Read the model definition and answer for the solid it produces. Units are mm, in the model's axes. A direction names the side the tool comes from. Coordinates: 2 decimals unless noted, no trailing zeros. Loops run counter-clockwise (first coordinate to the right, second up) from the corner with the lowest first, then second, coordinate; pieces in that order, holes last.
Q1. Straight lines are drawn through the part: line 1 (X direction, y = 2.35, z = 12); line 2 (Y direction, x = 15, z = -2.25); line 3 (X direction, y = 87.8, z = 0.25). For each, find the intervals that lie inside material, in ascending order.
Q2. The mould has two halves that part along Y. Classify faces 1 (the face through (-10, 2, 15)), 2 (the face through (-10, 0, 0)), 3 (the face through (-11.75, 85, -1)): pulls with the +Y half, pulls with the -Y half, needs draft (parallel to the pull), parting line crosses it, or undercut.
Q3. Section A-A (x = 14.5) is taken. Give the vertices of the cut face in (y, z), then the cut area to 3 significant figures.
Q4. Section D-D (x = -76.7) is taken. Give the vertices of the cut face in (y, z), then the cut area to 3 significant figures.
Q5. Flat-ended cylindrical pins translate along their axes: P1, Ø13.5, axis at x = 8.5, y = 77.5, coming from the +Z side; P2, Ø3, axis at x = 14.5, z = -12, coming from the -Y side; P3, Ø3, axis at y = 22.5, z = -1.5, coming from the -X side; P4, Ø5, axis at x = 16.5, z = 2.5, coming from the -Y side. Find the tip coordinate at first contact, or state that the pin passes through.
Q6. Section B-B (y = 63) is taken. Give the vertices of the cut face in (x, z), then the cut area to 3 significant figures.
Q7. Which of the six approach directions +Z, -Z, +X, -X, +Y, -Y give full straight-line access (tool end or side, diameter ignored) to faces 4 (the face through (23, 89.8, -1)), 5 (the face through (-10, 68, -12)), 6 (the face through (-11, 3, 7)), 7 (the face through (-9, 91, 6))?
Q8. Section C-C (z = 1.75) is taken. Give the vertices of the cut face in (x, y).
from build123d import *

# Parameters (mm, degrees)
SKETCH_1_W               = 126.3
SKETCH_1_H               = 42.9
SKETCH_1_W_2             = 2
SKETCH_1_W_3             = 62.15
EXTRUDE_6_DEPTH          = 15
SKETCH_2_W               = 62.15
SKETCH_2_H               = 42.9
CUT_EXTRUDE_1_DEPTH      = 23
SKETCH_4_W               = 10
SKETCH_4_H               = 40
CUT_EXTRUDE_2_DEPTH      = 159.899905601
CUT_EXTRUDE_3_DEPTH      = 119.456321064
CUT_EXTRUDE_3_DEPTH_BACK = 119.456321064
SKETCH_5_W               = 10
SKETCH_5_H               = 40
CUT_EXTRUDE_4_DEPTH      = 159.899905601
CUT_EXTRUDE_4_DEPTH_BACK = 159.899905601
SKETCH_6_W               = 9
SKETCH_6_H               = 46.7
SKETCH_7_W               = 14
SKETCH_7_H               = 11.9
CUT_EXTRUDE_5_DEPTH      = 23
SKETCH_9_R               = 1.6
CUT_EXTRUDE_6_DEPTH      = 10
CUT_EXTRUDE_7_DEPTH      = 159.899905601
CUT_EXTRUDE_7_DEPTH_BACK = 159.899905601
SKETCH_11_W              = 3
SKETCH_11_H              = 46.7
SKETCH_14_W              = 7
SKETCH_14_H              = 18
EXTRUDE_8_DEPTH          = 46.7
SKETCH_15_W              = 2.315581883
SKETCH_15_H              = 42.9
SKETCH_15_R              = 1.6
CUT_EXTRUDE_9_DEPTH      = 14
SKETCH_19_W              = 3
SKETCH_19_H              = 18
EXTRUDE_9_DEPTH          = 46.7
SKETCH_20_W              = 140.3
SKETCH_20_H              = 2
EXTRUDE_10_DEPTH         = 18
SKETCH_21_R              = 1.6
CUT_EXTRUDE_13_DEPTH     = 14
SKETCH_23_W              = 2
SKETCH_23_H              = 2
EXTRUDE_11_DEPTH         = 14


with BuildPart() as part:
    # 草图1 → 凸台-拉伸6 (new, symmetric)
    # profile 1 of 4: a face of its own
    with BuildSketch(Plane.XY):
        Polygon((-39.5, 0), (-39.5, 3), (-21.5, 3), (-21.5, 43), (-75.9, 43), (-75.9, 89.7), (54.4, 89.7), (54.4, 43), (0, 43), (0, 3), (18, 3), (18, 0), align=None)
        with Locations((-10.75, 66.35)):
            Rectangle(SKETCH_1_W, SKETCH_1_H, mode=Mode.SUBTRACT)
    # profile 2 of 4: a face of its own
    with BuildSketch(Plane.XY):
        with Locations((-10.75, 66.35)):
            Rectangle(SKETCH_1_W_2, SKETCH_1_H)
    # profile 3 of 4: a face of its own
    with BuildSketch(Plane.XY):
        with Locations((21.325, 66.35)):
            Rectangle(SKETCH_1_W_3, SKETCH_1_H)
    # profile 4 of 4: a face of its own
    with BuildSketch(Plane.XY):
        with Locations((-42.825, 66.35)):
            Rectangle(SKETCH_1_W_3, SKETCH_1_H)
    extrude(amount=EXTRUDE_6_DEPTH, both=True)

    # 草图2 → 切除-拉伸1 (cut)
    with BuildSketch(Plane.XY.offset(15)):
        with Locations((-42.825, 66.35)):
            Rectangle(SKETCH_2_W, SKETCH_2_H)
        with Locations((21.325, 66.35)):
            Rectangle(SKETCH_2_W, SKETCH_2_H)
    extrude(amount=-CUT_EXTRUDE_1_DEPTH, mode=Mode.SUBTRACT)

    # 草图4 → 切除-拉伸2 (cut, through all)
    with BuildSketch(Plane.ZY.offset(75.9)):
        with Locations((10, 23)):
            Rectangle(SKETCH_4_W, SKETCH_4_H)
    extrude(amount=-CUT_EXTRUDE_2_DEPTH, mode=Mode.SUBTRACT)

    # 草图5 → 切除-拉伸3 (cut, two sides: drawn at the far end of the back side and taken through both)
    with BuildSketch(Plane.ZY.offset(21.5).offset(-CUT_EXTRUDE_3_DEPTH_BACK)):
        with Locations((-10, 23)):
            Rectangle(SKETCH_5_W, SKETCH_5_H)
    extrude(amount=CUT_EXTRUDE_3_DEPTH + CUT_EXTRUDE_3_DEPTH_BACK, mode=Mode.SUBTRACT)

    # 草图6 → 切除-拉伸4 (cut, two sides: drawn at the far end of the back side and taken through both)
    with BuildSketch(Plane.ZY.offset(75.9).offset(-CUT_EXTRUDE_4_DEPTH_BACK)):
        with Locations((10.5, 66.35)):
            Rectangle(SKETCH_6_W, SKETCH_6_H)
    extrude(amount=CUT_EXTRUDE_4_DEPTH + CUT_EXTRUDE_4_DEPTH_BACK, mode=Mode.SUBTRACT)

    # 草图7 → 切除-拉伸5 (cut)
    with BuildSketch(Plane.ZY.offset(11.75)):
        with Locations((-1, 73.85)):
            Rectangle(SKETCH_7_W, SKETCH_7_H)
    extrude(amount=-CUT_EXTRUDE_5_DEPTH, mode=Mode.SUBTRACT)

    # 草图9 → 切除-拉伸6 (cut)
    with BuildSketch(Plane.XZ):
        with Locations(Location((-36, 12, 0), (0, 0, 270))):
            Circle(SKETCH_9_R)
        with Locations(Location((-36, -12, 0), (0, 0, 270))):
            Circle(SKETCH_9_R)
        with Locations(Location((14.5, 12, 0), (0, 0, 270))):
            Circle(SKETCH_9_R)
        with Locations(Location((14.5, -12, 0), (0, 0, 270))):
            Circle(SKETCH_9_R)
    extrude(amount=-CUT_EXTRUDE_6_DEPTH, mode=Mode.SUBTRACT)

    # 草图11 → 切除-拉伸7 (cut, two sides: drawn at the far end of the back side and taken through both)
    with BuildSketch(Plane.ZY.offset(75.9).offset(-CUT_EXTRUDE_7_DEPTH_BACK)):
        with Locations((-13.5, 66.35)):
            Rectangle(SKETCH_11_W, SKETCH_11_H)
    extrude(amount=CUT_EXTRUDE_7_DEPTH + CUT_EXTRUDE_7_DEPTH_BACK, mode=Mode.SUBTRACT)

    # 草图14 → 凸台-拉伸8 (add)
    with BuildSketch(Plane(origin=(0, 89.7, 0), x_dir=(1, 0, 0), z_dir=(0, 1, 0))):
        with Locations((57.9, 3)):
            Rectangle(SKETCH_14_W, SKETCH_14_H)
    extrude(amount=-EXTRUDE_8_DEPTH)

    # 草图15 → 切除-拉伸9 (cut)
    with BuildSketch(Plane.XY.offset(6)):
        with BuildLine():
            ThreePointArc((60.11573898, 44.9), (58.51573898, 46.5), (56.91573898, 44.9))
            ThreePointArc((56.91573898, 44.9), (58.51573898, 43.3), (60.11573898, 44.9))
        make_face()
        with Locations((53.557790942, 66.35)):
            Rectangle(SKETCH_15_W, SKETCH_15_H)
        Polygon((52.4, 44.9), (52.4, 87.8), (-9.75, 87.8), (-9.75, 79.8), (-11.75, 79.8), (-11.75, 87.8), (-73.9, 87.8), (-73.9, 44.9), (-11.75, 44.9), (-11.75, 67.9), (-9.75, 67.9), (-9.75, 44.9), align=None)
        with Locations((58.51385679, 87.8)):
            Circle(SKETCH_15_R)
    extrude(amount=-CUT_EXTRUDE_9_DEPTH, mode=Mode.SUBTRACT)

    # 草图19 → 凸台-拉伸9 (add)
    with BuildSketch(Plane(origin=(0, 89.7, 0), x_dir=(1, 0, 0), z_dir=(0, 1, 0))):
        with Locations((-77.4, 3)):
            Rectangle(SKETCH_19_W, SKETCH_19_H)
    extrude(amount=-EXTRUDE_9_DEPTH)

    # 草图20 → 凸台-拉伸10 (add)
    with BuildSketch(Plane.XY.offset(6)):
        with Locations((-8.75, 90.7)):
            Rectangle(SKETCH_20_W, SKETCH_20_H)
    extrude(amount=-EXTRUDE_10_DEPTH)

    # 草图21 → 切除-拉伸13 (cut)
    with BuildSketch(Plane.XY.offset(6)):
        with Locations((-76.7, 44.9)):
            Circle(SKETCH_21_R)
        Polygon((-73.9, 89.8), (-73.9, 87.8), (-11.75, 87.8), (54.715581883, 87.8), (54.715581883, 89.8), align=None)
        with Locations((-76.7, 87.8)):
            Circle(SKETCH_21_R)
    extrude(amount=-CUT_EXTRUDE_13_DEPTH, mode=Mode.SUBTRACT)

    # 草图23 → 凸台-拉伸11 (add)
    with BuildSketch(Plane.XY.offset(-8)):
        with Locations((-10.75, 88.8)):
            Rectangle(SKETCH_23_W, SKETCH_23_H)
    extrude(amount=EXTRUDE_11_DEPTH)


solid = part.part
Numbers:
1. line 1: x = -39.5 to -37.6, -34.4 to 12.9, 16.1 to 18
1. line 2: y = 0 to 3, 43 to 44.9, 89.8 to 91.7
1. line 3: x = -78.9 to -78.3, -75.1 to -73.9, -11.75 to -9.75, 54.72 to 56.91, 60.11 to 61.4
2. face 1: needs draft
2. face 2: pulls with the -Y half
2. face 3: undercut
3. outline: (0, -15) - (3, -15) - (3, -13.6) - (0, -13.6) - close; (0, -10.4) - (3, -10.4) - (3, 10.4) - (0, 10.4) - close; (0, 13.6) - (3, 13.6) - (3, 15) - (0, 15) - close; (43, -12) - (91.7, -12) - (91.7, 6) - (89.8, 6) - (89.8, -8) - (44.9, -8) - (44.9, 6) - (43, 6) - close
3. area: 319 mm2
4. outline: (43, -12) - (91.7, -12) - (91.7, 6) - (89.4, 6) - (89.4, -8) - (86.2, -8) - (86.2, 6) - (46.5, 6) - (46.5, -8) - (43.3, -8) - (43.3, 6) - (43, 6) - close
4. area: 787 mm2
5. P1: stops at z = -8
5. P2: stops at y = 43
5. P3: stops at x = -21.5
5. P4: stops at y = 0
6. outline: (-78.9, -12) - (61.4, -12) - (61.4, 6) - (54.72, 6) - (54.72, -8) - (-9.75, -8) - (-9.75, 6) - (-11.75, 6) - (-11.75, -8) - (-73.9, -8) - (-73.9, 6) - (-78.9, 6) - close
6. area: 753 mm2
7. face 4: +Z
7. face 5: -Z, +X, -X, +Y
7. face 6: none
7. face 7: +Z, +X, -X, +Y
8. outline: (-78.9, 43) - (-21.5, 43) - (-21.5, 3) - (-39.5, 3) - (-39.5, 0) - (18, 0) - (18, 3) - (0, 3) - (0, 43) - (61.4, 43) - (61.4, 91.7) - (-78.9, 91.7) - close; hole circle Ø3.2 at (-76.7, 44.9); hole circle Ø3.2 at (-76.7, 87.8); hole (-73.9, 44.9) - (-11.75, 44.9) - (-11.75, 67.9) - (-9.75, 67.9) - (-9.75, 44.9) - (54.72, 44.9) - (54.72, 89.8) - (-9.75, 89.8) - (-9.75, 79.8) - (-11.75, 79.8) - (-11.75, 89.8) - (-73.9, 89.8) - close; hole circle Ø3.2 at (58.51, 87.8); hole circle Ø3.2 at (58.52, 44.9)
